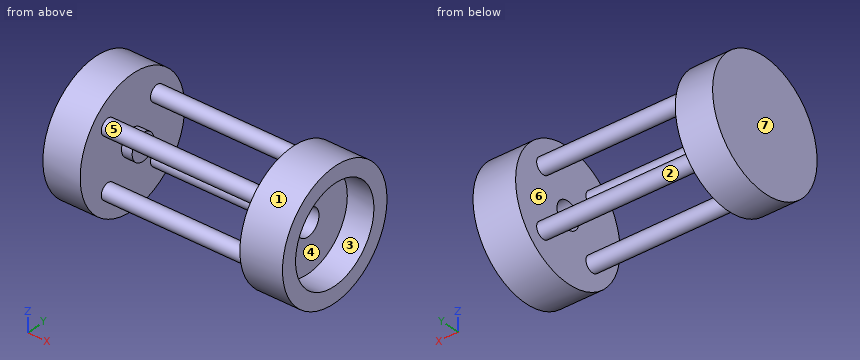
from build123d import *

# Parameters (mm, degrees)
F0_R      = 120
F1_DEPTH  = 70
F2_R      = 25
F3_DEPTH  = 20
F4_R      = 15
F5_DEPTH  = 300
F6_R      = 120
F7_DEPTH  = 80
F8_R      = 90
F9_DEPTH  = 50
F10_R     = 25
F11_DEPTH = 60


with BuildPart() as f1:
    # F0 (on Right) → F1 (new body)
    with BuildSketch(Plane.YZ):
        Circle(F0_R)
    extrude(amount=F1_DEPTH)

    # F2 (on face) → F3 (join)
    with BuildSketch(Plane.YZ.offset(70)):
        Circle(F2_R)
    extrude(amount=F3_DEPTH)

    # F4 (on face) → F5 (join)
    with BuildSketch(Plane.YZ.offset(70)):
        with Locations((-56.5685424949, -56.5685424949)):
            Circle(F4_R)
        with Locations((-56.5685424949, 56.5685424949)):
            Circle(F4_R)
        with Locations((56.5685424949, 56.5685424949)):
            Circle(F4_R)
        with Locations((56.5685424949, -56.5685424949)):
            Circle(F4_R)
    extrude(amount=F5_DEPTH)

    # F6 (on face) → F7 (join)
    with BuildSketch(Plane.YZ.offset(370)):
        Circle(F6_R)
    extrude(amount=F7_DEPTH)

    # F8 (on face) → F9 (cut)
    with BuildSketch(Plane.YZ.offset(450)):
        Circle(F8_R)
    extrude(amount=-F9_DEPTH, mode=Mode.SUBTRACT)

    # F10 (on face) → F11 (cut)
    with BuildSketch(Plane.YZ.offset(400)):
        Circle(F10_R)
    extrude(amount=-F11_DEPTH, mode=Mode.SUBTRACT)


solid = f1.part
Work out the finished part from the listing and answer in its coordinate system (mm). Face numbers are marked on the shaded views. A direction names the side the tool comes from. Round coordinates to 2 decimals unless told otherwise and drop trailing zeros. Loops run counter-clockwise (first coordinate to the right, second up) from the corner with the lowest first, then second, coordinate; pieces in that order, holes last. Notation, with made-up numbers: (63, -1) - (108, -1) arc R13 ccw to (108, 23) - close; hole circle Ø10 at (23.25, 20). An arc over 180 degrees is marked (long way). Use one line per item in the form item = value. Start each with the question number.
(1) Find section C-C on z = 33. Determine the outline of the cut face in (x, y), and give its area (3 significant figures).
(2) Determine the mould class of the marked faces 4, 5, 6 and 7 for opening direction X: +X half, -X half, draft (parallel to the pull), parting line (faces both ways), or undercut.
(3) Find section A-A on y = 0. Determine the outline of the cut face in (x, z), and give its area (3 significant figures).
(4) Find section D-D on y = 83.5. Determine the outline of the cut face in (x, z), and give its area (3 significant figures).
(5) Consider line 1 (X direction, y = 39, z = -88); line 2 (Z direction, x = 385.75, y = 0); line 3 (Z direction, x = 428, y = 0). Determine where each line is inside the solid, lowest interval first.
(6) Flat-ended cylindrical pins translate along their axes: P1, Ø1.5, axis at x = 293.5, y = -49, coming from the -Z side; P2, Ø4, axis at x = 102.5, y = 72, coming from the -Z side; P3, Ø1.5, axis at x = 47, z = -10.5, coming from the +Y side. Find the tip coordinate at first contact, or state that the pin passes through.
(7) Which of the six approach directions +Z, -Z, +X, -X, +Y, -Y give full straight-line access (tool end or side, diameter ignored) to the marked faces 1, 2 and 3?
Answer list:
q1.outline = (0, -115.37) - (70, -115.37) - (70, 115.37) - (0, 115.37) - close; (370, -115.37) - (450, -115.37) - (450, -83.73) - (400, -83.73) - (400, 83.73) - (450, 83.73) - (450, 115.37) - (370, 115.37) - close
q1.area = 26,200 mm^2
q2.face_4 = +X half
q2.face_5 = undercut
q2.face_6 = undercut
q2.face_7 = -X half
q3.outline = (0, -120) - (70, -120) - (70, -25) - (90, -25) - (90, 25) - (70, 25) - (70, 120) - (0, 120) - close; (370, -120) - (450, -120) - (450, -90) - (400, -90) - (400, -25) - (370, -25) - close; (370, 25) - (400, 25) - (400, 90) - (450, 90) - (450, 120) - (370, 120) - close
q3.area = 26,500 mm^2
q4.outline = (0, -86.18) - (70, -86.18) - (70, 86.18) - (0, 86.18) - close; (370, -86.18) - (450, -86.18) - (450, -33.58) - (400, -33.58) - (400, 33.58) - (450, 33.58) - (450, 86.18) - (370, 86.18) - close
q4.area = 22,500 mm^2
q5.line_1 = 0 to 70, 370 to 450
q5.line_2 = -120 to -25, 25 to 120
q5.line_3 = -120 to -90, 90 to 120
q6.P1 = -69.93
q6.P2 = -63.25
q6.P3 = 119.6
q7.face_1 = +X, -X
q7.face_2 = none
q7.face_3 = +X
